```python
from build123d import *

# Parameters (mm, degrees)
BOSS_EXTRUDE1_DEPTH = 5
CUT_EXTRUDE1_DEPTH  = 43.772012023
FILLET1_R           = 2.54
SKETCH3_W           = 20
SKETCH3_H           = 7.5
BOSS_EXTRUDE2_DEPTH = 34.4
SKETCH4_W           = 4.75
SKETCH4_H           = 1.7
BOSS_EXTRUDE3_DEPTH = 15
CUT_EXTRUDE2_DEPTH  = 71.664569081
FILLET2_R           = 2.54


with BuildPart() as part:
    # Sketch1 → Boss-Extrude1 (new body)
    with BuildSketch(Plane(origin=(0, 0, 0), x_dir=(1, 0, 0), z_dir=(0, 1, 0))):
        Polygon((-29.999623956, -29.926382831), (30.000376044, -29.926382831), (30.000376044, -9.926382831), (10.000376044, -9.926382831), (10.000376044, 10.073617169), (30.000376044, 10.073617169), (30.000376044, 30.073617169), (-29.999623956, 30.073617169), (-29.999623956, 10.073617169), (-9.999623956, 10.073617169), (-9.999623956, -9.926382831), (-29.999623956, -9.926382831), align=None)
    extrude(amount=BOSS_EXTRUDE1_DEPTH)

    # Sketch2 → Cut-Extrude1 (cut, through all)
    with BuildSketch(Plane(origin=(0, 5, 0), x_dir=(1, 0, 0), z_dir=(0, 1, 0))):
        with BuildLine():
            Line((-18.549247911, 18.573617169), (18.55, 18.573617169))
            ThreePointArc((18.55, 18.573617169), (19.575304833, 18.998312337), (20, 20.023617169))
            Line((20, 20.023617169), (20, 20.123617169))
            ThreePointArc((20, 20.123617169), (19.575304833, 21.148922002), (18.55, 21.573617169))
            Line((18.55, 21.573617169), (-18.549247911, 21.573617169))
            ThreePointArc((-18.549247911, 21.573617169), (-19.574552744, 21.148922002), (-19.999247911, 20.123617169))
            Line((-19.999247911, 20.123617169), (-19.999247911, 20.023617169))
            ThreePointArc((-19.999247911, 20.023617169), (-19.574552744, 18.998312337), (-18.549247911, 18.573617169))
        make_face()
        with BuildLine():
            Line((-18.549623956, -21.426382831), (18.550376044, -21.426382831))
            ThreePointArc((18.550376044, -21.426382831), (19.575680877, -21.001687663), (20.000376044, -19.976382831))
            Line((20.000376044, -19.976382831), (20.000376044, -19.876382831))
            ThreePointArc((20.000376044, -19.876382831), (19.575680877, -18.851077998), (18.550376044, -18.426382831))
            Line((18.550376044, -18.426382831), (-18.549623956, -18.426382831))
            ThreePointArc((-18.549623956, -18.426382831), (-19.574928788, -18.851077998), (-19.999623956, -19.876382831))
            Line((-19.999623956, -19.876382831), (-19.999623956, -19.976382831))
            ThreePointArc((-19.999623956, -19.976382831), (-19.574928788, -21.001687663), (-18.549623956, -21.426382831))
        make_face()
    extrude(amount=-CUT_EXTRUDE1_DEPTH, mode=Mode.SUBTRACT)

    # Fillet1
    fillet1_edges = [part.edges().sort_by_distance(p)[0] for p in [
        (-29.999623956, 2.5, -10.073617169),
        (-29.999623956, 2.5, -30.073617169),
        (30.000376044, 2.5, -30.073617169),
        (30.000376044, 2.5, -10.073617169),
        (10.000376044, 2.5, -10.073617169),
        (10.000376044, 2.5, 9.926382831),
        (30.000376044, 2.5, 9.926382831),
        (30.000376044, 2.5, 29.926382831),
        (-29.999623956, 2.5, 29.926382831),
        (-29.999623956, 2.5, 9.926382831),
        (-9.999623956, 2.5, 9.926382831),
        (-9.999623956, 2.5, -10.073617169),
    ]]
    fillet(fillet1_edges, radius=FILLET1_R)

    # Sketch3 → Boss-Extrude2 (add)
    with BuildSketch(Plane(origin=(0, 5, 0), x_dir=(1, 0, 0), z_dir=(0, 1, 0))):
        Rectangle(SKETCH3_W, SKETCH3_H)
    extrude(amount=BOSS_EXTRUDE2_DEPTH)

    # Sketch4 → Boss-Extrude3 (add)
    with BuildSketch(Plane(origin=(0, 39.4, 0), x_dir=(1, 0, 0), z_dir=(0, 1, 0))):
        Polygon((10, -3.75), (10, -0.85), (5.25, -0.85), (-5.25, -0.85), (-10, -0.85), (-10, -3.75), align=None)
        with Locations((7.625, 0)):
            Rectangle(SKETCH4_W, SKETCH4_H)
        Polygon((5.25, 0.85), (10, 0.85), (10, 3.75), (-10, 3.75), (-10, 0.85), (-5.25, 0.85), align=None)
        with Locations((-7.625, 0)):
            Rectangle(SKETCH4_W, SKETCH4_H)
    extrude(amount=BOSS_EXTRUDE3_DEPTH)

    # Sketch5 → Cut-Extrude2 (cut, through all)
    with BuildSketch(Plane(origin=(0, 0, -3.75), x_dir=(-1, 0, 0), z_dir=(0, 0, -1))):
        with BuildLine():
            Line((-1.21, 41), (1.21, 41))
            ThreePointArc((1.21, 41), (3.006051224, 41.743948776), (3.75, 43.54))
            Line((3.75, 43.54), (3.75, 46.46))
            ThreePointArc((3.75, 46.46), (3.006051224, 48.256051224), (1.21, 49))
            Line((1.21, 49), (-1.21, 49))
            ThreePointArc((-1.21, 49), (-3.006051224, 48.256051224), (-3.75, 46.46))
            Line((-3.75, 46.46), (-3.75, 43.54))
            ThreePointArc((-3.75, 43.54), (-3.006051224, 41.743948776), (-1.21, 41))
        make_face()
    extrude(amount=-CUT_EXTRUDE2_DEPTH, mode=Mode.SUBTRACT)

    # Fillet2
    fillet2_edges = [part.edges().sort_by_distance(p)[0] for p in [
        (0.000188022, 5, 3.75),
        (0.000188022, 5, -3.75),
        (-10, 54.4, 0),
        (10, 54.4, 0),
    ]]
    fillet(fillet2_edges, radius=FILLET2_R)


solid = part.part
```
Build history of the part. All positions in model axes, mm. A direction names the side the tool comes from. Round coordinates to 2 decimals unless told otherwise and drop trailing zeros. Order: outer loops, then holes, each group sorted by start corner. A loop starts at its lowest first (then second) coordinate and runs counter-clockwise, first axis right, second up. Notation, with made-up numbers: (24.5, -9.75) - (57.5, -9.75) arc R26 ccw to (57.5, 23.25) - close; hole circle Ø5 at (5, 0). An arc over 180 degrees is marked (long way). Use a Markdown table: item, result.
1) Saw through at D-D on x = -9. Write the cut outline in (y, z), and give its area (3 significant figures).
Recorded:
| item | result |
|---|---|
| outline | (0, -30.07) - (5, -30.07) - (5, -21.57) - (0, -21.57) - close; (0, -18.57) - (5, -18.57) - (5, -6.29) arc R2.54 cw to (7.54, -3.75) - (53.88, -3.75) - (53.88, 3.75) - (7.54, 3.75) arc R2.54 cw to (5, 6.29) - (5, 18.43) - (0, 18.43) - close; (0, 21.43) - (5, 21.43) - (5, 29.93) - (0, 29.93) - close |
| area | 639 mm² |
2) Pull direction Z, two halves, no side cores. Call faces 1 (the face through (-9.236, 53.676, 0.053)), 2 (the face through (29.24, 2.54, -10.8)), 3 (the face through (0.14, 5.764, -4.474)): pulls with the +Z half, pulls with the -Z half, needs draft (parallel to the pull), parting line crosses it, or undercut.
Recorded:
| item | result |
|---|---|
| face 1 | needs draft |
| face 2 | undercut |
| face 3 | pulls with the -Z half |
3) Tool access for faces 4 (the face through (0, 5, -7)), 5 (the face through (2.986, 48.276, 2.28)), 6 (the face through (0, 29, -3.75)): list every direction of +Z, -Z, +X, -X, +Y, -Y with a clear straight run to the whole face (end or side of a thin tool).
Recorded:
| item | result |
|---|---|
| face 4 | +X, -X, +Y |
| face 5 | +Z, -Z |
| face 6 | -Z, +X, -X, +Y |
4) Wall check: L1, parallel to Z at x = 9, y = 47; L2, parallel to Y at x = -12, z = 11. Give the ranges that are in metal, low to high.
Recorded:
| item | result |
|---|---|
| L1 | z = -3.75 to 3.75 |
| L2 | y = 0 to 5 |
5) Saw through at A-A on x = 14. Write the cut outline in (y, z).
Recorded:
| item | result |
|---|---|
| outline | (0, -30.07) - (5, -30.07) - (5, -21.57) - (0, -21.57) - close; (0, -18.57) - (5, -18.57) - (5, -10.07) - (0, -10.07) - close; (0, 9.93) - (5, 9.93) - (5, 18.43) - (0, 18.43) - close; (0, 21.43) - (5, 21.43) - (5, 29.93) - (0, 29.93) - close |
6) Saw through at C-C on y = 48. Write the cut outline in (x, z), and give its area (3 significant figures).
Recorded:
| item | result |
|---|---|
| outline | (-10, -3.75) - (-3.23, -3.75) - (-3.23, -0.85) - (-5.25, -0.85) - (-5.25, 0.85) - (-3.23, 0.85) - (-3.23, 3.75) - (-10, 3.75) - close; (3.23, -3.75) - (10, -3.75) - (10, 3.75) - (3.23, 3.75) - (3.23, 0.85) - (5.25, 0.85) - (5.25, -0.85) - (3.23, -0.85) - close |
| area | 94.7 mm² |
7) Flat gauge pins, fed straight in: pin 1 Ø10 at (x, y) = (13, 37) entering from +Z; pin 2 Ø2.5 at (y, z) = (2, 0.5) entering from +X; pin 3 Ø12 at (x, z) = (23.5, -12.5) entering from +Y; pin 4 Ø5 at (x, z) = (17, -7.5) entering from +Y. Where does each tip first touch, or does it go through?
Recorded:
| item | result |
|---|---|
| pin 1 | stops at z = 3.75 |
| pin 2 | stops at x = 10 |
| pin 3 | stops at y = 5 |
| pin 4 | passes through |
8) Saw through at B-B on x = 26.5. Write the cut outline in (y, z), and give its area (3 significant figures).
Recorded:
| item | result |
|---|---|
| outline | (0, -30.07) - (5, -30.07) - (5, -10.07) - (0, -10.07) - close; (0, 9.93) - (5, 9.93) - (5, 29.93) - (0, 29.93) - close |
| area | 200 mm² |
